from build123d import *

# Parameters (mm, degrees)
F1_DEPTH = 5
F2_DEPTH = 5
F3_DEPTH = 5


# Not quite as in the source:
# - a feature names something its author has since deleted; it is built from what else it names


with BuildPart() as f1:
    # F0 (on Front) → F1 (new body)
    with BuildSketch(Plane.XZ):
        Polygon((-50.9245342757, -5.52e-08), (-100.9245342757, -5.52e-08), (-100.9245342757, -7), (-105.9245342757, -7), (-105.924534339, -22), (-100.9245342757, -22), (-100.9245342757, -38), (-105.9245342757, -38), (-105.924534339, -53), (-100.9245342757, -53), (-100.9245342757, -60.0000000552), (-98.924534339, -60.0000000552), (-98.924534339, -65.0000000552), (-83.924534339, -65), (-83.924534339, -60.0000000552), (-73.924534339, -60.0000000552), (-73.924534339, -65.0000000552), (-58.924534339, -65), (-58.924534339, -60.0000000552), (-42.9245342757, -60.0000000552), (-42.9245342757, -65.0000000552), (-27.9245342757, -65.0000000552), (-27.9245342757, -60.0000000552), (-17.9245342757, -60.0000000552), (-17.9245342757, -65.0000000552), (-2.9245342757, -65.0000000552), (-2.9245342757, -60.0000000552), (-0.9245342757, -60.0000000552), (-0.9245342757, -53.0000000552), (4.0754657243, -53.0000000552), (4.0754657243, -38.0000000552), (-0.9245342757, -38.0000000552), (-0.9245342757, -22), (4.0754657243, -22), (4.075465661, -7), (-0.9245342757, -7), (-0.9245342757, -5.52e-08), align=None)
    extrude(amount=F1_DEPTH)

    # F0 (on Front) → F2 (join)
    with BuildSketch(Plane.XZ):
        with BuildLine():
            Line((-105.9245342757, -5.52e-08), (-100.9245342757, -5.52e-08))
            Line((-100.9245342757, -5.52e-08), (-50.9245342757, -5.52e-08))
            Line((-50.9245342757, -5.52e-08), (-0.9245342757, -5.52e-08))
            Line((-0.9245342757, -5.52e-08), (4.0754657243, -5.52e-08))
            Line((4.0754657243, -5.52e-08), (4.0754657243, 49.9999999448))
            ThreePointArc((4.0754657243, 49.9999999448), (2.6109996302, 53.5355338508), (-0.9245342757, 54.9999999448))
            Line((-0.9245342757, 54.9999999448), (-100.9245342757, 54.9999999448))
            ThreePointArc((-100.9245342757, 54.9999999448), (-104.4600681817, 53.5355338508), (-105.9245342757, 49.9999999448))
            Line((-105.9245342757, 49.9999999448), (-105.9245342757, -5.52e-08))
        make_face()
    extrude(amount=F2_DEPTH)

    # F0 (on Front) → F3 (join)
    with BuildSketch(Plane.XZ):
        with BuildLine():
            Line((-105.9245342757, -5.52e-08), (-100.9245342757, -5.52e-08))
            Line((-100.9245342757, -5.52e-08), (-50.9245342757, -5.52e-08))
            Line((-50.9245342757, -5.52e-08), (-0.9245342757, -5.52e-08))
            Line((-0.9245342757, -5.52e-08), (4.0754657243, -5.52e-08))
            Line((4.0754657243, -5.52e-08), (4.0754657243, 49.9999999448))
            ThreePointArc((4.0754657243, 49.9999999448), (2.6109996302, 53.5355338508), (-0.9245342757, 54.9999999448))
            Line((-0.9245342757, 54.9999999448), (-100.9245342757, 54.9999999448))
            ThreePointArc((-100.9245342757, 54.9999999448), (-104.4600681817, 53.5355338508), (-105.9245342757, 49.9999999448))
            Line((-105.9245342757, 49.9999999448), (-105.9245342757, -5.52e-08))
        make_face()
    extrude(amount=F3_DEPTH)


solid = f1.part
Can you work these out from the model? Positions are in its coordinate system, mm. A direction names the side the tool comes from. Coordinates: 2 decimals unless noted, no trailing zeros. Write each loop counter-clockwise with the first axis right and the second up, starting at its lowest first coordinate (ties: lowest second). Pieces come first, ordered by that corner, then holes. Notation, with made-up numbers: (-21, -29) -> (-9, -29) arc R16 cw to (-9, -10) -> close; hole circle Ø8 at (-29, -22.5). An arc over 180 degrees is marked (long way). Write each question's results on one line, items separated by ' | '. Start each with the question number.
Item 1: Thinking about a two-plate mould opening in X: for faces 6 (the flat face through (-0.925, -2, -30)), 7 (the flat face through (-52, 0, -4)), 8 (the flat face through (-79, -2, -60)), which applies, released by +X, released by -X, zero draft, split by the parting line, or undercut?
Item 2: On a 3-axis mill with a long thin cutter (end or side, diameter ignored), from which of +Z, -Z, +X, -X, +Y, -Y can I reach the whole of each face in a straight line? I mean faces 1 (the flat face through (2, -2, -22)), 2 (the flat face through (-73.925, -2, -62)), 3 (the flat face through (-0.925, -2, -57)), 4 (the flat face through (-67, -2, -65)), 5 (the flat face through (-100.925, -2, -30)). Say none if no direction works.
Item 3: I'm going to push flat-ended pins straight in: P1, Ø2.5, axis at y = -2, z = -57.5, coming from the -X side; P2, Ø1.5, axis at y = -2.5, z = -62.5, coming from the +X side; P3, Ø1.5, axis at y = -3, z = -5, coming from the +X side. Where does each tip first touch, or does it pass through?
Item 4: Please list where these lines run through material, in increasing order: probe 1 along Z at (x, y) = (-22, -1.2); probe 2 along X at (y, z) = (-2.6, -28).
Item 5: If we section it at A-A, the plane z = -55: Write out the boundary of the cut face in (x, y), and give its area (3 significant figures).
Answer block:
1) face 6: released by +X | face 7: zero draft | face 8: undercut
2) face 1: +X, +Y, -Y | face 2: -Z, +Y, -Y | face 3: -Z, +X, +Y, -Y | face 4: -Z, +X, -X, +Y, -Y | face 5: -X, +Y, -Y
3) P1: x = -100.92 | P2: x = -2.92 | P3: x = -0.92
4) probe 1: -60 to 55 | probe 2: -100.92 to -0.92
5) outline: (-100.92, -5) -> (-0.92, -5) -> (-0.92, 0) -> (-100.92, 0) -> close | area: 500 mm²
